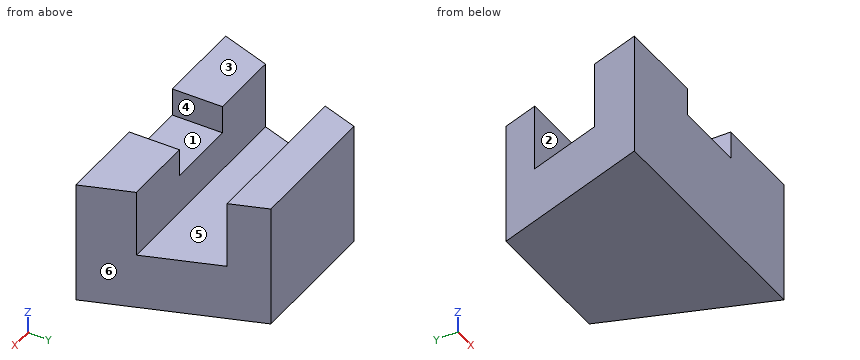
```python
from build123d import *

# Parameters (mm, degrees)
BOSS_EXTRUDE1_DEPTH     = 44
CUT_EXTRUDE1_DEPTH      = 86.586213843
CUT_EXTRUDE1_DEPTH_BACK = 86.586213843
SKETCH2_W               = 24
SKETCH2_H               = 27
SKETCH3_W               = 26
SKETCH3_H               = 18
CUT_EXTRUDE2_DEPTH      = 10


with BuildPart() as part:
    # Sketch1 → Boss-Extrude1 (new body)
    with BuildSketch(Plane.XY):
        Polygon((-45, 0), (45, 0), (25, 58), (-25, 58), align=None)
    extrude(amount=BOSS_EXTRUDE1_DEPTH)

    # Sketch2 → Cut-Extrude1 (cut, two sides: drawn at the far end of the back side and taken through both)
    with BuildSketch(Plane(origin=(0, 0, 0), x_dir=(0, 0, -1), z_dir=(1, 0, 0)).offset(-CUT_EXTRUDE1_DEPTH_BACK)):
        with Locations((-32, 31.5)):
            Rectangle(SKETCH2_W, SKETCH2_H)
    extrude(amount=CUT_EXTRUDE1_DEPTH + CUT_EXTRUDE1_DEPTH_BACK, mode=Mode.SUBTRACT)

    # Sketch3 → Cut-Extrude2 (cut)
    with BuildSketch(Plane.XY.offset(44)):
        with Locations((0, 9)):
            Rectangle(SKETCH3_W, SKETCH3_H)
    extrude(amount=-CUT_EXTRUDE2_DEPTH, mode=Mode.SUBTRACT)


solid = part.part
```
Design review of the part built by this model. Coordinates are the model's own, in mm. Face numbers are marked on the shaded views. A direction names the side the tool comes from. Coordinates: 2 decimals unless noted, no trailing zeros. Order: outer loops, then holes, each group sorted by start corner. A loop starts at its lowest first (then second) coordinate and runs counter-clockwise, first axis right, second up. Notation, with made-up numbers: M -20,64.25 L -6,64.25 A16 ccw -6,85.25 Z; hole C -2.75,-17.75 d6. An arc over 180 degrees is marked long. Answer as a JSON object with one key per item and string values. Group by question number.
1) Wall thickness on L1, parallel to Z at x = 13, y = 44.5; L2, parallel to Y at x = -16, z = 37.5; L3, parallel to X at y = 6, z = 36: over which ranges is each line inside the solid? List them lowest first.
2) Add section A-A, the plane z = 27. Write out the cut boundary in (x, y), then the cut area to 3 significant figures.
3) Add section C-C, the plane y = 5. Write out the cut boundary in (x, z), then the cut area to 3 significant figures.
4) Add section B-B, the plane x = -6. Write out the cut boundary in (y, z), then the cut area to 3 significant figures.
5) Add section D-D, the plane x = -32. Write out the cut boundary in (y, z).
6) Mouldability with a two-part tool opening along X and no side actions: class the marked faces 4, 5 and 6 as pulls with the +X half, pulls with the -X half, needs draft (parallel to the pull), parting line crosses it, or undercut.
7) Tool access review of the marked faces 1, 2 and 3: name each direction out of +Z, -Z, +X, -X, +Y, -Y from which nothing blocks a thin tool from reaching the whole face with its end or side.
8) For pin 1 (9 mm diameter, centred on x = -2, y = 4.5, fed in from +Z); pin 2 (11 mm diameter, centred on y = 10, z = 37, fed in from +X); pin 3 (8 mm diameter, centred on x = -27.5, y = 37.5, fed in from +Z), all flat-tipped, find the tip position at first contact; note any pin that passes through.
Computed values:
{
 "1": {"L1": "z = 0 to 20", "L2": "y = 0 to 18, 45 to 58", "L3": "x = -42.93 to -13, 13 to 42.93"},
 "2": {"outline": "M -45,0 L 45,0 L 38.79,18 L -38.79,18 Z; M -29.48,45 L 29.48,45 L 25,58 L -25,58 Z", "area": "2,220 mm^2"},
 "3": {"outline": "M -43.28,0 L 43.28,0 L 43.28,44 L 13,44 L 13,34 L -13,34 L -13,44 L -43.28,44 Z", "area": "3,550 mm^2"},
 "4": {"outline": "M 0,0 L 58,0 L 58,44 L 45,44 L 45,20 L 18,20 L 18,34 L 0,34 Z", "area": "1,720 mm^2"},
 "5": {"outline": "M 0,0 L 37.7,0 L 37.7,20 L 18,20 L 18,44 L 0,44 Z"},
 "6": {"face 4": "undercut", "face 5": "needs draft", "face 6": "pulls with the +X half"},
 "7": {"face 1": "+Z, -Y", "face 2": "+Z, +X, -X", "face 3": "+Z, +X, -X, +Y, -Y"},
 "8": {"pin 1": "stops at z = 34", "pin 2": "stops at x = 43.45", "pin 3": "stops at z = 20"}
}
